Geometry: final body of the model. Coordinates: model frame, mm. A direction names the side the tool comes from. Round coordinates to 2 decimals unless told otherwise and drop trailing zeros. Loops run counter-clockwise (first coordinate to the right, second up) from the corner with the lowest first, then second, coordinate; pieces in that order, holes last. Notation, with made-up numbers: (-32.5, 82.25) - (-14.5, 82.25) arc R22 cw to (-14.5, 115.25) - close; hole circle Ø1 at (22, 62). An arc over 180 degrees is marked (long way). Answer as a JSON object with one key per item and string values. Group by question number.
Item 1: Line query: line 1 (Z direction, x = -64, y = 41); line 2 (Y direction, x = -75.5, z = 39.5); line 3 (Y direction, x = -8.5, z = 55). Output: solid intervals per line, ascending.
Item 2: Reachability of faces 1 (the face through (-40, 27, 25)), 2 (the face through (-108.313, 24, 12)) from +Z, -Z, +X, -X, +Y, -Y: full face, straight path, thin tool, end or side. Return the list, or none.
Item 3: Draft query along Y for faces 3 (the face through (31.687, 24, 12)), 4 (the face through (-75.165, 58.676, 61.975)), 5 (the face through (-1.6, 38, 63)). Return one class per face: released by +Y, released by -Y, zero draft, split by the parting line, or undercut.
Item 4: Section D-D (y = 85). Return the cut outline in (x, z), plus the area to 3 significant figures.
Item 5: Section B-B (y = 6.5). Return the cut outline in (x, z).
Item 6: Section C-C (z = 38). Return the cut outline in (x, y).
Item 7: Section A-A (x = -5). Return the cut outline in (y, z).
Item 8: First-contact query: pin 1 (12 mm diameter, centred on x = -39.5, y = -29.5, fed in from +Z); pin 2 (1.5 mm diameter, centred on x = -50, z = 80.5, fed in from -Y); pin 3 (1 mm diameter, centred on y = 22, z = 59.5, fed in from -X). Flat tips, straight axial feed; report the tip coordinate or a pass-through.
```python
from build123d import *

# Parameters (mm, degrees)
F0_W     = 140
F0_H     = 140
F1_DEPTH = 25
F2_R     = 50
F3_DEPTH = 75
F4_R     = 40
F5_DEPTH = 75


with BuildPart() as f1:
    # F0 (on Top) → F1 (new body)
    with BuildSketch(Plane.XY):
        with Locations((-38.313064, 24.884112)):
            Rectangle(F0_W, F0_H)
    extrude(amount=F1_DEPTH)

    # F2 (on face) → F3 (join)
    with BuildSketch(Plane.XY.offset(25)):
        with Locations((-38.313064, 24.884112)):
            Circle(F2_R)
    extrude(amount=F3_DEPTH)

    # F4 (on face) → F5 (cut)
    with BuildSketch(Plane.XY.offset(100)):
        with Locations((-39.742772, 25.948399)):
            Circle(F4_R)
    extrude(amount=-F5_DEPTH, mode=Mode.SUBTRACT)


solid = f1.part
```
Values:
{
 "1": {"line 1": "z = 0 to 25", "line 2": "y = -8.54 to 8.02, 43.88 to 58.31", "line 3": "y = -15.26 to 0.97, 50.93 to 65.02"},
 "2": {"face 1": "+Z", "face 2": "+Z, -Z, -X, +Y, -Y"},
 "3": {"face 3": "zero draft", "face 4": "split by the parting line", "face 5": "undercut"},
 "4": {"outline": "(-108.31, 0) - (31.69, 0) - (31.69, 25) - (-108.31, 25) - close", "area": "3,500 mm^2"},
 "5": {"outline": "(-108.31, 0) - (31.69, 0) - (31.69, 25) - (8.18, 25) - (8.18, 100) - (-4.79, 100) - (-4.79, 25) - (-74.7, 25) - (-74.7, 100) - (-84.81, 100) - (-84.81, 25) - (-108.31, 25) - close"},
 "6": {"outline": "circle Ø100 at (-38.31, 24.88); hole circle Ø80 at (-39.74, 25.95)"},
 "7": {"outline": "(-45.12, 0) - (94.88, 0) - (94.88, 25) - (62.17, 25) - (62.17, 100) - (45.77, 100) - (45.77, 25) - (6.13, 25) - (6.13, 100) - (-12.4, 100) - (-12.4, 25) - (-45.12, 25) - close"},
 "8": {"pin 1": "stops at z = 100", "pin 2": "stops at y = -23.91", "pin 3": "stops at x = -88.26"}
}
